The listing builds one solid part. Answer for the finished solid, in the listing's coordinates (mm). A direction names the side the tool comes from. Round coordinates to 2 decimals unless told otherwise and drop trailing zeros. Loops run counter-clockwise (first coordinate to the right, second up) from the corner with the lowest first, then second, coordinate; pieces in that order, holes last. Notation, with made-up numbers: (17.25, 6) -> (41.25, 6) arc R20 ccw to (41.25, 19) -> close; hole circle Ø11 at (75, -13). An arc over 180 degrees is marked (long way). Write each question's results on one line, items separated by ' | '. Start each with the question number.
Autodesk Inventor part; units mm, degrees
ref_plane "YZ Plane" through (0, 0, 0) normal (1, 0, 0) x (0, 1, 0)
ref_plane "XZ Plane" through (0, 0, 0) normal (0, 1, 0) x (-1, 0, 0)
ref_plane "XY Plane" through (0, 0, 0) normal (0, 0, 1) x (1, 0, 0)
sketch "Sketch1" plane through (0, 0, 0) normal (0, 1, 0) x (-1, 0, 0)
  line L0 (38.5, 80) -> (-38.5, 80)
  line L1 (-38.5, 80) -> (-38.5, -80)
  line L2 (-38.5, -80) -> (38.5, -80)
  line L3 (38.5, -80) -> (38.5, 80)
  line L4 (38.5, 0) -> (-38.5, 0) construction
  line L5 (0, 80) -> (0, -80) construction
  line L6 (-22.5, -80) -> (22.5, -80)
  line L7 (22.5, -80) -> (22.5, -75)
  line L8 (22.5, -75) -> (-22.5, -75)
  line L9 (-22.5, -75) -> (-22.5, -80)
  point P0 (0, 0)
  point P1 (0, 0)
  dimension "d0" = 77
  dimension "d1" = 160
  dimension "d64" = 45
  dimension "d65" = 5
extrude "Extrusion1" add sketch "Sketch1" along normal blind 5 contours L3 L2 L7 L8 L9 L1 L0
fillet "Fillet1" radius 5 4 edges at (-38.5, 2.5, 80) (38.5, 2.5, 80) (38.5, 2.5, -80) (-38.5, 2.5, -80)
sketch "Sketch3" plane through (0, 5, 0) normal (0, 1, 0) x (1, 0, 0)
  line L0 (33.5, 80) -> (-33.5, 80) construction
  line L1 (-30.75, -72) -> (-30.75, 75) construction
  line L2 (-30.75, 75) -> (30.75, 75) construction
  line L3 (30.75, 75) -> (30.75, -72) construction
  line L4 (30.75, -72) -> (-30.75, -72) construction
  line L5 (0, 112) -> (0, -112) construction
  line L6 (-33.5, -80) -> (33.5, -80)
  line L7 (38.5, -75) -> (38.5, 75)
  line L8 (-38.5, 75) -> (-38.5, -75)
  point P0 (0, 0)
  point P1 (0, -72)
  point P2 (0, -80)
  dimension "d15" = 147
  dimension "d18" = 8
  dimension "d56" = 61.5
hole "Brass stands" at (-30.75, 5, 72) at (30.75, 5, 72) at (30.75, 5, -75) at (-30.75, 5, -75) direction (0, -1, 0) diameter 3.4 end through all
sketch "Sketch5" plane through (0, 5, 0) normal (0, 1, 0) x (1, 0, 0)
  line L0 (-23, -5) -> (23, -5) construction
  line L1 (23, -5) -> (23, 25) construction
  line L2 (23, 25) -> (-23, 25) construction
  line L3 (-23, 25) -> (-23, -5) construction
  line L4 (-23, -5) -> (23, 25) construction
  line L5 (23, -5) -> (-23, 25) construction
  line L6 (0, 112) -> (0, -112) construction
  line L7 (33.5, 80) -> (-33.5, 80) construction
  point P0 (0, 0)
  point P1 (0, 10)
  point P2 (0, 10)
  point P3 (-23, 25)
  point P4 (23, 25)
  dimension "d31" = 30
  dimension "d32" = 46
  dimension "d33" = 55
hole "Battery mount" at (-23, 5, 5) at (-23, 5, -25) at (23, 5, -25) at (23, 5, 5) direction (0, -1, 0) diameter 3.4 end through all
sketch "Sketch7" plane through (0, 5, 0) normal (0, 1, 0) x (1, 0, 0)
  line L0 (7.5, 24) -> (-7.5, 24) construction
  line L1 (-7.5, 24) -> (-7.5, 10.5) construction
  line L2 (-7.5, 10.5) -> (7.5, 10.5) construction
  line L3 (7.5, 10.5) -> (7.5, 24) construction
  line L4 (7.5, 24) -> (-7.5, 10.5) construction
  line L5 (-7.5, 24) -> (7.5, 10.5) construction
  line L6 (33.5, 80) -> (22.5, 80) construction
  line L7 (38.5, -75) -> (38.5, 75) construction
  line L8 (22.5, 75) -> (-22.5, 75) construction
  line L9 (0, 112) -> (0, -112) construction
  point P0 (0, 0)
  point P1 (0, 17.25)
  point P2 (54.473, 10.5)
  point P3 (0, 24)
  point P4 (0, 17.25)
  dimension "d66" = 13.5
  dimension "d67" = 15
  dimension "d71" = 51
hole "pi cam" at (7.5, 5, -24) at (7.5, 5, -10.5) at (54.473, 5, -10.5) at (-7.5, 5, -24) at (-7.5, 5, -10.5) direction (0, -1, 0) diameter 3.4 end through all
sketch "Sketch8" plane through (0, 5, 0) normal (0, 1, 0) x (1, 0, 0)
  circle A0 centre (-7.5, 24) radius 1.7
  circle A1 centre (7.5, 10.5) radius 1.7
  circle A2 centre (7.5, 24) radius 1.7
  circle A3 centre (-7.5, 10.5) radius 1.7
  circle A4 centre (23, 25) radius 1.7
  circle A5 centre (-23, -5) radius 1.7
  circle A6 centre (-23, 25) radius 1.7
  circle A7 centre (23, -5) radius 1.7
  circle A8 centre (30.75, 75) radius 1.7
  circle A9 centre (-30.75, -72) radius 1.7
  circle A10 centre (30.75, -72) radius 1.7
  circle A11 centre (-30.75, 75) radius 1.7
  arc A12 (-33.5, 80) -> (-38.5, 75) centre (-33.5, 75) ccw
  line L0 (-38.5, 75) -> (-38.5, -75)
  arc A13 (-38.5, -75) -> (-33.5, -80) centre (-33.5, -75) ccw
  line L1 (-33.5, -80) -> (33.5, -80)
  arc A14 (33.5, -80) -> (38.5, -75) centre (33.5, -75) ccw
  line L2 (38.5, -75) -> (38.5, 75)
  arc A15 (38.5, 75) -> (33.5, 80) centre (33.5, 75) ccw
  line L3 (33.5, 80) -> (22.5, 80)
  line L4 (22.5, 80) -> (22.5, 75)
  line L5 (22.5, 75) -> (-22.5, 75)
  line L6 (-22.5, 75) -> (-22.5, 80)
  line L7 (-22.5, 80) -> (-33.5, 80)
  line L8 (30.75, 0) -> (-18.25, 0) construction
  line L9 (-18.25, 0) -> (-18.25, -58) construction
  line L10 (-18.25, -58) -> (30.75, -58) construction
  line L11 (30.75, -58) -> (30.75, 0) construction
  line L12 (30.75, 0) -> (-18.25, -58) construction
  line L13 (-18.25, 0) -> (30.75, -58) construction
  point P0 (0, 0)
  point P1 (6.25, -29)
  dimension "d79" = 49
  dimension "d80" = 58
  dimension "d81" = 22
  dimension "d82" = 7.75
hole "raspberry pi" at (30.75, 5, 0) at (30.75, 5, 58) at (-18.25, 5, 58) at (-18.25, 5, 0) direction (0, -1, 0) diameter 3.4 end through all
sketch "buck convertor" plane through (0, 5, 0) normal (0, 1, 0) x (1, 0, 0)
  line L0 (38.5, -75) -> (38.5, 75)
  circle A0 centre (-18.25, -58) radius 1.7
  circle A1 centre (30.75, 0) radius 1.7
  circle A2 centre (30.75, -58) radius 1.7
  circle A3 centre (-18.25, 0) radius 1.7
  circle A4 centre (-7.5, 24) radius 1.7
  circle A5 centre (7.5, 10.5) radius 1.7
  circle A6 centre (7.5, 24) radius 1.7
  circle A7 centre (-7.5, 10.5) radius 1.7
  circle A8 centre (23, 25) radius 1.7
  circle A9 centre (-23, -5) radius 1.7
  circle A10 centre (-23, 25) radius 1.7
  circle A11 centre (23, -5) radius 1.7
  circle A12 centre (30.75, 75) radius 1.7
  circle A13 centre (-30.75, -72) radius 1.7
  circle A14 centre (30.75, -72) radius 1.7
  circle A15 centre (-30.75, 75) radius 1.7
  arc A16 (-33.5, 80) -> (-38.5, 75) centre (-33.5, 75) ccw
  line L1 (-38.5, 75) -> (-38.5, -75)
  arc A17 (-38.5, -75) -> (-33.5, -80) centre (-33.5, -75) ccw
  line L2 (-33.5, -80) -> (33.5, -80)
  arc A18 (33.5, -80) -> (38.5, -75) centre (33.5, -75) ccw
  line L3 (38.5, -75) -> (38.5, 75)
  arc A19 (38.5, 75) -> (33.5, 80) centre (33.5, 75) ccw
  line L4 (33.5, 80) -> (22.5, 80)
  line L5 (22.5, 80) -> (22.5, 75)
  line L6 (22.5, 75) -> (-22.5, 75)
  line L7 (-22.5, 75) -> (-22.5, 80)
  line L8 (-22.5, 80) -> (-33.5, 80)
  line L9 (30.75, 70) -> (-30.75, 70) construction
  line L10 (-30.75, 70) -> (-30.75, 38) construction
  line L11 (-30.75, 38) -> (30.75, 38) construction
  line L12 (30.75, 38) -> (30.75, 70) construction
  line L13 (30.75, 70) -> (-30.75, 38) construction
  line L14 (-30.75, 70) -> (30.75, 38) construction
  line L15 (0, 113.4497) -> (0, -113.4497)
  point P0 (0, 0)
  point P1 (0, 54)
  point P2 (0, 54)
  dimension "d90" = 32
  dimension "d98" = 10
hole "Hole7" at (30.75, 5, -38) at (-30.75, 5, -38) at (30.75, 5, -70) at (-30.75, 5, -70) direction (0, -1, 0) diameter 3.4 end through all
properties part number "Top plate" material "PBT Plastic"
Item 1: Determine the mould class of faces 3 (the flat face through (-38.5, 2, -1)), 4 (the cylindrical face through (-30.8, 2.5, -76.7)), 5 (the flat face through (28, 2, -80)) for opening direction X: +X half, -X half, draft (parallel to the pull), parting line (faces both ways), or undercut.
Item 2: The part is cut by section D-D, the plane y = 0.75. Give the number of separate pieces and of enclosed holes in the cut face, plus the area to 3 significant figures.
Item 3: The part is cut by section A-A, the plane z = 0. Give the vertices of the cut face in (x, y).
Item 4: The part is cut by section C-C, the plane x = -18.25. Give the vertices of the cut face in (y, z).
Item 5: The part is cut by section B-B, the plane x = 30.75. Give the vertices of the cut face in (y, z), plus the area to 3 significant figures.
Item 6: For faces 1 (the flat face through (0, 2, -75)), 2 (the cylindrical face through (9, 2.5, -9.7)), determine the directions among +Z, -Z, +X, -X, +Y, -Y from which every point of the face is accessible in a straight line to the end or side of a thin tool.
Item 7: Straight lines are drawn through the part: L1, parallel to X at y = 3.8, z = 5; L2, parallel to Z at x = 23, y = 0.8; L3, parallel to X at y = 2.4, z = 0. For each, find the intervals that lie inside material, in ascending order. Write a range as [from, to].
Item 8: Each of these flat-tipped pins is pushed along its axis until it touches: pin 1 Ø1.5 at (y, z) = (2.5, -78.5) entering from -X; pin 2 Ø2.5 at (x, z) = (-23, 5) entering from -Y. Where does it stop, or does it pass through?
Report:
1) face 3: -X half | face 4: undercut | face 5: draft
2) separate pieces: 1 | enclosed holes: 20 | area: 11,900 mm2
3) outline: (-38.5, 0) -> (-19.95, 0) -> (-19.95, 5) -> (-38.5, 5) -> close; (-16.55, 0) -> (29.05, 0) -> (29.05, 5) -> (-16.55, 5) -> close; (32.45, 0) -> (38.5, 0) -> (38.5, 5) -> (32.45, 5) -> close
4) outline: (0, -75) -> (5, -75) -> (5, -1.7) -> (0, -1.7) -> close; (0, 1.7) -> (5, 1.7) -> (5, 56.3) -> (0, 56.3) -> close; (0, 59.7) -> (5, 59.7) -> (5, 80) -> (0, 80) -> close
5) outline: (0, -80) -> (5, -80) -> (5, -76.7) -> (0, -76.7) -> close; (0, -73.3) -> (5, -73.3) -> (5, -71.7) -> (0, -71.7) -> close; (0, -68.3) -> (5, -68.3) -> (5, -39.7) -> (0, -39.7) -> close; (0, -36.3) -> (5, -36.3) -> (5, -1.7) -> (0, -1.7) -> close; (0, 1.7) -> (5, 1.7) -> (5, 56.3) -> (0, 56.3) -> close; (0, 59.7) -> (5, 59.7) -> (5, 70.3) -> (0, 70.3) -> close; (0, 73.7) -> (5, 73.7) -> (5, 80) -> (0, 80) -> close | area: 698 mm2
6) face 1: -Z, +Y, -Y | face 2: +Y, -Y
7) L1: x = [-38.5, -24.7], [-21.3, 21.3], [24.7, 38.5] | L2: z = [-80, -26.7], [-23.3, 3.3], [6.7, 80] | L3: x = [-38.5, -19.95], [-16.55, 29.05], [32.45, 38.5]
8) pin 1: stops at x = -37.68 | pin 2: passes through
